Job drawing, mm, ordinate dimensions from the low corner. One solid piece. A direction names the side the tool comes from. Coordinates: 2 decimals unless noted, no trailing zeros. Write each loop counter-clockwise with the first axis right and the second up, starting at its lowest first coordinate (ties: lowest second). Pieces come first, ordered by that corner, then holes. Notation, with made-up numbers: (75, -26.5) -> (113, -26.5) arc R26 ccw to (113, -6.5) -> close; hole circle Ø11 at (5, 60). An arc over 180 degrees is marked (long way). One line per question, with ' | ' between items. Start each with the question number.
Item 1: Pin check, flat tips, straight feed: pin 1 (3 mm diameter, centred on y = 12.5, z = 35.5, fed in from -X); pin 2 (12.5 mm diameter, centred on y = 11, z = 36.5, fed in from +X); pin 3 (2 mm diameter, centred on x = 59.5, z = 46.5, fed in from +Y). Stop position of each tip, or through.
Item 2: Saw through at C-C (x = 60.5). List the corners of the cut face in (y, z), and give its area (3 significant figures).
Item 3: Saw through at D-D (y = 20.25). List the corners of the cut face in (x, z).
Item 4: Saw through at B-B (z = 22). List the corners of the cut face in (x, y).
Item 5: Two-plate mould, pull along Z, no slides. Class the marked faces 3, 4, 5 and 6: pulls with the +Z half, pulls with the -Z half, needs draft (parallel to the pull), parting line crosses it, or undercut.
Item 6: 3-axis set-ups, long thin cutter, end or side, ignore diameter. For the marked faces 1 and 2: which of +Z, -Z, +X, -X, +Y, -Y reach the whole face in a straight line?
Item 7: Saw through at A-A (x = 16). List the corners of the cut face in (y, z).
Item 8: Probe probe 1 along Z at (x, y) = (3.5, 1.55); probe 2 along X at (y, z) = (1.8, 3.5); probe 3 along Z at (x, y) = (11.5, 16.75). List the from-to ranges inside material, lowest first. Write a range as [from, to].
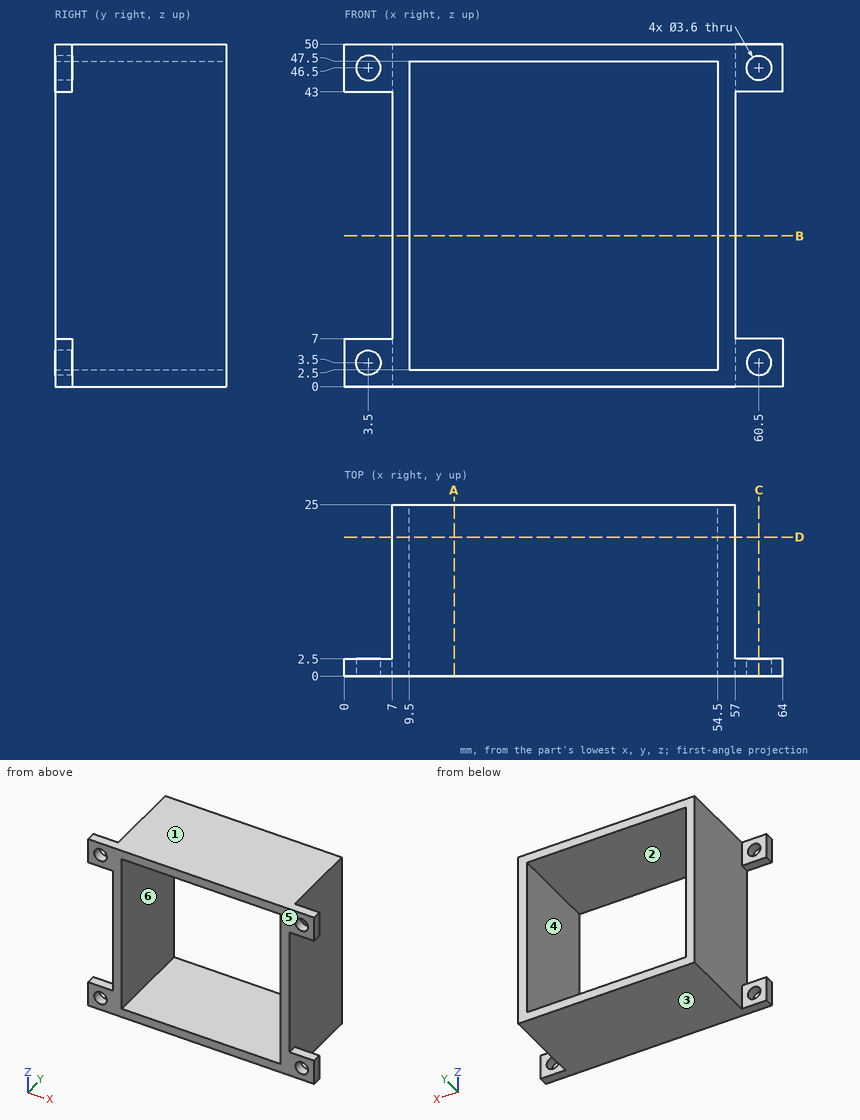
From the geometry:
1) pin 1: x = 7 | pin 2: x = 57 | pin 3: y = 2.5
2) outline: (0, 0) -> (2.5, 0) -> (2.5, 1.7) -> (0, 1.7) -> close; (0, 5.3) -> (2.5, 5.3) -> (2.5, 7) -> (0, 7) -> close; (0, 43) -> (2.5, 43) -> (2.5, 44.7) -> (0, 44.7) -> close; (0, 48.3) -> (2.5, 48.3) -> (2.5, 50) -> (0, 50) -> close | area: 17.0 mm2
3) outline: (7, 0) -> (57, 0) -> (57, 50) -> (7, 50) -> close; hole (9.5, 2.5) -> (54.5, 2.5) -> (54.5, 47.5) -> (9.5, 47.5) -> close
4) outline: (7, 0) -> (9.5, 0) -> (9.5, 25) -> (7, 25) -> close; (54.5, 0) -> (57, 0) -> (57, 25) -> (54.5, 25) -> close
5) face 3: pulls with the -Z half | face 4: undercut | face 5: needs draft | face 6: undercut
6) face 1: +Z, +X, -X, +Y, -Y | face 2: +Y, -Y
7) outline: (0, 0) -> (25, 0) -> (25, 2.5) -> (0, 2.5) -> close; (0, 47.5) -> (25, 47.5) -> (25, 50) -> (0, 50) -> close
8) probe 1: [0, 1.7], [5.3, 7], [43, 44.7], [48.3, 50] | probe 2: [0, 1.7], [5.3, 9.5], [54.5, 58.7], [62.3, 64] | probe 3: [0, 2.5], [47.5, 50]
